Part print with two shaded views. Sizes in mm from the minimum x, y, z corner. Coordinates: 2 decimals unless noted, no trailing zeros. Loops run counter-clockwise (first coordinate to the right, second up) from the corner with the lowest first, then second, coordinate; pieces in that order, holes last. Notation, with made-up numbers: (83, -24.5) -> (114, -24.5) arc R23 ccw to (114, -9.5) -> close; hole circle Ø5 at (7, 71). An arc over 180 degrees is marked (long way). Return JSON: item names as keys, results as strings. Group by question number.
(1) Probe L1, parallel to X at y = 8.5, z = 15.5 (3 decimals). List the from-to ranges inside material, lowest first.
(2) Saw through at B-B on z = 14. Write the cut outline in (x, y) (3 decimals), then the cut area to 3 significant figures.
(3) Saw through at A-A on y = 7.75. Write the cut outline in (x, z) (3 decimals), then the cut area to 3 significant figures.
(4) Flat gauge pins, fed straight in: pin 1 Ø8 at (y, z) = (10, 10) entering from -X (3 decimals); pin 2 Ø8 at (x, y) = (677.5, 11) entering from -Z (3 decimals); pin 3 Ø2 at (y, z) = (8, 9) entering from +X. Where does each tip first touch, or does it go through?
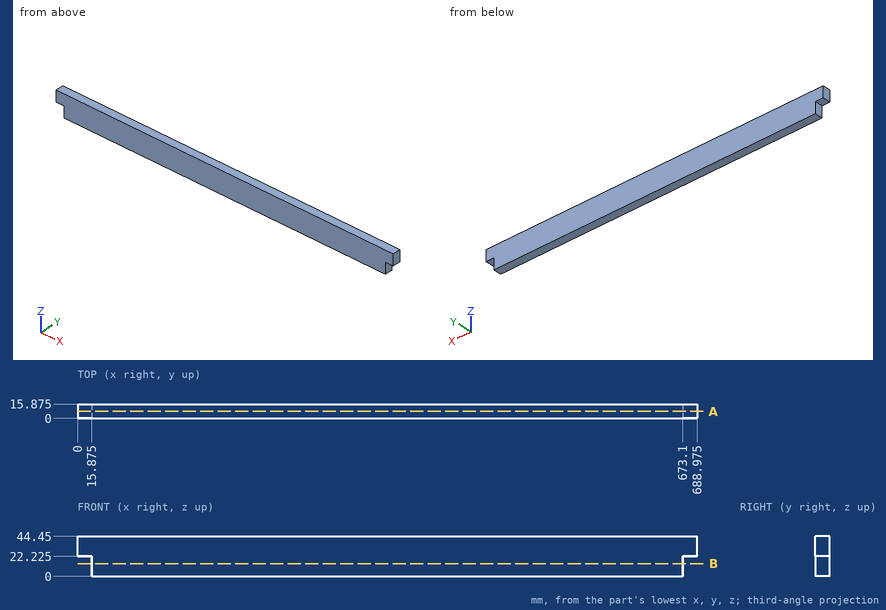
Geometry results:
{
 "1": {"L1": "15.875 to 673.1"},
 "2": {"outline": "(15.875, 0) -> (673.1, 0) -> (673.1, 15.875) -> (15.875, 15.875) -> close", "area": "10,400 mm²"},
 "3": {"outline": "(0, 22.225) -> (15.875, 22.225) -> (15.875, 0) -> (673.1, 0) -> (673.1, 22.225) -> (688.975, 22.225) -> (688.975, 44.45) -> (0, 44.45) -> close", "area": "29,900 mm²"},
 "4": {"pin 1": "x = 15.875", "pin 2": "z = 22.225", "pin 3": "x = 673.1"}
}
